```python
from build123d import *

# Parameters (mm, degrees)
F0_R     = 6.25
F1_DEPTH = 12.5
F3_DEPTH = 19
F6_DEPTH = 90.8642213825


with BuildPart() as f1:
    # F0 (on Top) → F1 (new body)
    with BuildSketch(Plane.XY):
        with BuildLine():
            ThreePointArc((6.5, 0), (0, -6.5), (-6.5, 0))
            Line((-6.5, 0), (-6.5, 13))
            Line((-6.5, 13), (-32, 13))
            ThreePointArc((-32, 13), (-45, 0), (-32, -13))
            Line((-32, -13), (-19, -13))
            Line((-19, -13), (-19, -77))
            Line((-19, -77), (-32, -77))
            ThreePointArc((-32, -77), (-45, -90), (-32, -103))
            Line((-32, -103), (32, -103))
            ThreePointArc((32, -103), (45, -90), (32, -77))
            Line((32, -77), (19, -77))
            Line((19, -77), (19, -13))
            Line((19, -13), (32, -13))
            ThreePointArc((32, -13), (45, 0), (32, 13))
            Line((32, 13), (6.5, 13))
            Line((6.5, 13), (6.5, 0))
        make_face()
        with Locations((-32, -90)):
            Circle(F0_R, mode=Mode.SUBTRACT)
        with Locations((32, -90)):
            Circle(F0_R, mode=Mode.SUBTRACT)
        with Locations((-32, 0)):
            Circle(F0_R, mode=Mode.SUBTRACT)
        with Locations((32, 0)):
            Circle(F0_R, mode=Mode.SUBTRACT)
    extrude(amount=F1_DEPTH)

    # F2 (on Right) → F3 (join, symmetric)
    with BuildSketch(Plane.YZ):
        Polygon((-103, 12.5), (-77, 12.5), (-53.5025253169, 12.5), (-78.2512626585, 37.2487373415), align=None)
    extrude(amount=F3_DEPTH, both=True)

    # F4 (on face) → F5 (join, up to the next surface of F1)
    with BuildSketch(Plane(origin=(0, -57.75, 57.75), x_dir=(1, 0, 0), z_dir=(0, -0.7071067812, 0.7071067812))):
        with BuildLine():
            ThreePointArc((19, -28.9931636974), (0, -9.9931636974), (-19, -28.9931636974))
            Line((-19, -28.9931636974), (-13.143277803, -28.9931636974))
            Line((-13.143277803, -28.9931636974), (-12.6607489396, -27.5080925584))
            ThreePointArc((-12.6607489396, -27.5080925584), (-14.2658477444, -24.3579087818), (-11.1156639678, -22.752809977))
            Line((-11.1156639678, -22.752809977), (-9.0817816001, -16.4931636974))
            Line((-9.0817816001, -16.4931636974), (-2.5, -16.4931636974))
            ThreePointArc((-2.5, -16.4931636974), (0, -13.9931636974), (2.5, -16.4931636974))
            Line((2.5, -16.4931636974), (9.0817816001, -16.4931636974))
            Line((9.0817816001, -16.4931636974), (11.1156639678, -22.752809977))
            ThreePointArc((11.1156639678, -22.752809977), (13.3576695844, -23.1079087818), (14.3882064537, -25.1304512677))
            ThreePointArc((14.3882064537, -25.1304512677), (13.9107489396, -26.5999143984), (12.6607489396, -27.5080925584))
            Line((12.6607489396, -27.5080925584), (13.143277803, -28.9931636974))
            Line((13.143277803, -28.9931636974), (19, -28.9931636974))
        make_face()
        with BuildLine():
            Line((-12.6607489396, -27.5080925584), (-13.143277803, -28.9931636974))
            Line((-13.143277803, -28.9931636974), (-7.5, -28.9931636974))
            ThreePointArc((-7.5, -28.9931636974), (0, -21.4931636974), (7.5, -28.9931636974))
            Line((7.5, -28.9931636974), (13.143277803, -28.9931636974))
            Line((13.143277803, -28.9931636974), (12.6607489396, -27.5080925584))
            ThreePointArc((12.6607489396, -27.5080925584), (9.510565163, -25.9029937536), (11.1156639678, -22.752809977))
            Line((11.1156639678, -22.752809977), (9.0817816001, -16.4931636974))
            Line((9.0817816001, -16.4931636974), (2.5, -16.4931636974))
            ThreePointArc((2.5, -16.4931636974), (0, -18.9931636974), (-2.5, -16.4931636974))
            Line((-2.5, -16.4931636974), (-9.0817816001, -16.4931636974))
            Line((-9.0817816001, -16.4931636974), (-11.1156639678, -22.752809977))
            ThreePointArc((-11.1156639678, -22.752809977), (-9.8656639678, -23.660988137), (-9.3882064537, -25.1304512677))
            ThreePointArc((-9.3882064537, -25.1304512677), (-10.418743323, -27.1529937536), (-12.6607489396, -27.5080925584))
        make_face()
        with BuildLine():
            ThreePointArc((7.5, -28.9931636974), (0, -21.4931636974), (-7.5, -28.9931636974))
            Line((-7.5, -28.9931636974), (7.5, -28.9931636974))
        make_face()
    extrude(until=Until.NEXT, dir=(0, 0.7071067812, -0.7071067812))

    # F4 (on face) → F6 (cut, through all)
    with BuildSketch(Plane(origin=(0, -57.75, 57.75), x_dir=(1, 0, 0), z_dir=(0, -0.7071067812, 0.7071067812))):
        with BuildLine():
            Line((2.5, -16.4931636974), (-2.5, -16.4931636974))
            ThreePointArc((-2.5, -16.4931636974), (0, -18.9931636974), (2.5, -16.4931636974))
        make_face()
        with BuildLine():
            ThreePointArc((2.5, -16.4931636974), (0, -13.9931636974), (-2.5, -16.4931636974))
            Line((-2.5, -16.4931636974), (2.5, -16.4931636974))
        make_face()
        with BuildLine():
            Line((11.1156639678, -22.752809977), (12.6607489396, -27.5080925584))
            ThreePointArc((12.6607489396, -27.5080925584), (13.9107489396, -26.5999143984), (14.3882064537, -25.1304512677))
            ThreePointArc((14.3882064537, -25.1304512677), (13.3576695844, -23.1079087818), (11.1156639678, -22.752809977))
        make_face()
        with BuildLine():
            ThreePointArc((11.1156639678, -22.752809977), (9.510565163, -25.9029937536), (12.6607489396, -27.5080925584))
            Line((12.6607489396, -27.5080925584), (11.1156639678, -22.752809977))
        make_face()
        with BuildLine():
            ThreePointArc((-11.1156639678, -22.752809977), (-14.2658477444, -24.3579087818), (-12.6607489396, -27.5080925584))
            Line((-12.6607489396, -27.5080925584), (-11.1156639678, -22.752809977))
        make_face()
        with BuildLine():
            Line((-11.1156639678, -22.752809977), (-12.6607489396, -27.5080925584))
            ThreePointArc((-12.6607489396, -27.5080925584), (-10.418743323, -27.1529937536), (-9.3882064537, -25.1304512677))
            ThreePointArc((-9.3882064537, -25.1304512677), (-9.8656639678, -23.660988137), (-11.1156639678, -22.752809977))
        make_face()
        with BuildLine():
            Line((-5.3247731677, -40.5753392578), (-9.3698581396, -37.6364129963))
            ThreePointArc((-9.3698581396, -37.6364129963), (-8.8167787844, -41.128418613), (-5.3247731677, -40.5753392578))
        make_face()
        with BuildLine():
            ThreePointArc((-4.8473156537, -39.1058761271), (-6.5747731677, -36.7282348363), (-9.3698581396, -37.6364129963))
            Line((-9.3698581396, -37.6364129963), (-5.3247731677, -40.5753392578))
            ThreePointArc((-5.3247731677, -40.5753392578), (-4.9696743629, -39.878418613), (-4.8473156537, -39.1058761271))
        make_face()
        with BuildLine():
            ThreePointArc((9.8473156537, -39.1058761271), (9.7249569444, -38.3333336411), (9.3698581396, -37.6364129963))
            Line((9.3698581396, -37.6364129963), (5.3247731677, -40.5753392578))
            ThreePointArc((5.3247731677, -40.5753392578), (8.1198581396, -41.4835174178), (9.8473156537, -39.1058761271))
        make_face()
        with BuildLine():
            Line((5.3247731677, -40.5753392578), (9.3698581396, -37.6364129963))
            ThreePointArc((9.3698581396, -37.6364129963), (5.8778525229, -37.0833336411), (5.3247731677, -40.5753392578))
        make_face()
    extrude(amount=-F6_DEPTH, mode=Mode.SUBTRACT)


solid = f1.part
```
Could you check a few things on this model? Use its own coordinates, in mm. A direction names the side the tool comes from. Round coordinates to 2 decimals unless told otherwise and drop trailing zeros. Loops run counter-clockwise (first coordinate to the right, second up) from the corner with the lowest first, then second, coordinate; pieces in that order, holes last.
Q1. I want a section at C-C (x = -21.5). Write out the boundary of the cut face in (y, z), and give its area (3 significant figures).
Q2. I want a section at B-B (x = -1). Write out the boundary of the cut face in (y, z).
Q3. For P1, Ø10, axis at y = -62, z = 13, coming from the +X side; P2, Ø14, axis at y = 7, z = 9, coming from the +X side; P3, Ø18.5, axis at y = -37.5, z = 17, coming from the -X side; P4, Ø8, axis at x = 25.5, y = -87.5, coming from the +Z side, each with a flat end and sliding along its axis, tell me the tip position at first contact or that it passes through.
Q4. Thinking about a two-plate mould opening in Y: for faces 6 (the flat face through (6.5, 7, 6)), 7 (the cylindrical face through (0.1, -6.5, 6.2)), 8 (the cylindrical face through (45, -90, 6)), which applies, pulls with the +Y half, pulls with the -Y half, needs draft (parallel to the pull), parting line crosses it, or undercut?
Q5. On a 3-axis mill with a long thin cutter (end or side, diameter ignored), from which of +Z, -Z, +X, -X, +Y, -Y can I reach the whole of each face in a straight line? I mean faces 1 (the flat face through (-0.3, -83.6, 31.9)), 2 (the flat face through (26, -77, 6)), 3 (the flat face through (-26, -13, 6)), 4 (the flat face through (26, -93, 12.5)), 5 (the flat face through (-6.5, 6, 6)). Say none if no direction works.
Q6. Please list where these lines run through material, in increasing order: L1, parallel to Y at x = 32, z = 10; L2, parallel to Y at x = -21.5, z = 11; L3, parallel to Y at x = -6, z = 13.
Q7. I want a section at A-A (y = -90). Write out the boundary of the cut face in (x, z), and give its area (3 significant figures).
Answer below:
1. outline: (-103, 0) - (-77, 0) - (-77, 12.5) - (-103, 12.5) - close; (-13, 0) - (13, 0) - (13, 12.5) - (-13, 12.5) - close
1. area: 650 mm2
2. outline: (-103, 0) - (-26.57, 0) - (-71.03, 44.47) - (-103, 12.5) - close; (-67.79, 47.71) - (-20.08, 0) - (-6.42, 0) - (-6.42, 12.5) - (-26.67, 12.5) - (-64.83, 50.67) - close
3. P1: stops at x = 19
3. P2: stops at x = 45
3. P3: stops at x = -19
3. P4: stops at z = 12.5
4. face 6: needs draft
4. face 7: pulls with the +Y half
4. face 8: undercut
5. face 1: +Z, +X, -X, -Y
5. face 2: +Z, -Z, +X
5. face 3: +Z, -Z, -X
5. face 4: +Z, +X, +Y, -Y
5. face 5: +Z, -Z, +Y
6. L1: y = -103 to -96.25, -83.75 to -77, -13 to -6.25, 6.25 to 13
6. L2: y = -103 to -77, -13 to 13
6. L3: y = -102.5 to -71.28, -65.33 to -28.51
7. outline: (-45, 0) - (-38.25, 0) - (-38.25, 12.5) - (-45, 12.5) - close; (-25.75, 0) - (25.75, 0) - (25.75, 12.5) - (19, 12.5) - (19, 25.5) - (-19, 25.5) - (-19, 12.5) - (-25.75, 12.5) - close; (38.25, 0) - (45, 0) - (45, 12.5) - (38.25, 12.5) - close
7. area: 1,310 mm2
